```python
from build123d import *

# Parameters (mm, degrees)
CYLINDER1054_R           = 1
CYLINDER1054_DEPTH       = 5
CYLINDER1055_R           = 1
CYLINDER1055_DEPTH       = 5
BOX258_W                 = 36
BOX258_H                 = 16
BOX258_DEPTH             = 1.5
PAD042_DEPTH             = 3
CLONE020_PLACEMENT_ANGLE = -90


with BuildPart() as cylinder1062:
    # Cylinder1054 → Cylinder1054 (new body)
    with BuildSketch(Plane(origin=(33, 3, 0), x_dir=(1, 0, 0), z_dir=(0, 0, 1))):
        Circle(CYLINDER1054_R)
    extrude(amount=CYLINDER1054_DEPTH)


with BuildPart() as fusion151:
    # Cylinder1055 → Cylinder1055 (new body)
    with BuildSketch(Plane(origin=(33, 13, 0), x_dir=(1, 0, 0), z_dir=(0, 0, 1))):
        Circle(CYLINDER1055_R)
    extrude(amount=CYLINDER1055_DEPTH)

    # Fusion151: union Cylinder1062
    add(cylinder1062.part)


with BuildPart() as cut:
    # Box258 → Box258 (new body)
    with BuildSketch(Plane.XY):
        with Locations((18, 8)):
            Rectangle(BOX258_W, BOX258_H)
    extrude(amount=BOX258_DEPTH)

    # Cut: cut Fusion151
    add(fusion151.part, mode=Mode.SUBTRACT)


with BuildPart() as obj1:
    # Sketch067 → Pad042 (new body, symmetric)
    with BuildSketch(Plane(origin=(13, 8, 1.5), x_dir=(0, 0, 1), z_dir=(0, -1, 0))):
        Polygon((0, 0), (10, 0), (10, 3.8), (1.85, 3.8), (1.85, 8.8), (10, 8.8), (10, 12.6), (0, 12.6), align=None)
    extrude(amount=PAD042_DEPTH, both=True)

    # Fusion152: union Cut
    add(cut.part)


with BuildPart() as obj1_1:
    # Clone020 placement: moved
    add(obj1.part.moved(Location((-8, 61.0689, 26.1))).rotate(Axis((-8, 61.0689, 26.1), (0, 0, 1)), CLONE020_PLACEMENT_ANGLE))


solid = obj1_1.part
```
Work out the finished part from the listing and answer in its coordinate system (mm). A direction names the side the tool comes from. Coordinates: 2 decimals unless noted, no trailing zeros. Loops run counter-clockwise (first coordinate to the right, second up) from the corner with the lowest first, then second, coordinate; pieces in that order, holes last. Notation, with made-up numbers: (39.5, -5) - (70.5, -5) arc R23 ccw to (70.5, 24) - close; hole circle Ø3 at (2.25, -37). An arc over 180 degrees is marked (long way). Use a Markdown table: item, result.
Item 1: Find section D-D, the plane y = 57.5. Determine the outline of the cut face in (x, z), and give its area (3 significant figures).
Evaluation:
| item | result |
|---|---|
| outline | (-8, 26.1) - (8, 26.1) - (8, 27.6) - (3, 27.6) - (3, 37.6) - (-3, 37.6) - (-3, 27.6) - (-8, 27.6) - close |
| area | 84.0 mm2 |
Item 2: Find section A-A, the plane z = 31.25. Determine the outline of the cut face in (x, y).
Evaluation:
| item | result |
|---|---|
| outline | (-3, 48.07) - (3, 48.07) - (3, 51.87) - (-3, 51.87) - close; (-3, 56.87) - (3, 56.87) - (3, 60.67) - (-3, 60.67) - close |
Item 3: Given pin 1 Ø3 at (x, z) = (1.5, 31.5) entering from -Y; pin 2 Ø2.5 at (x, y) = (-5, 28.07) entering from +Z; pin 3 Ø3 at (x, z) = (-0.5, 34) entering from +Y; pin 4 Ø4 at (x, y) = (-0.5, 55.5) entering from +Z, each flat-ended and moving along its own axis, determine where each tip first touches the part or whether it passes through.
Evaluation:
| item | result |
|---|---|
| pin 1 | stops at y = 48.07 |
| pin 2 | stops at z = 27.6 |
| pin 3 | stops at y = 60.67 |
| pin 4 | stops at z = 37.6 |
Item 4: The mould has two halves that part along Y. Classify faces 5 (the flat face through (0, 54, 29.45)), 6 (the flat face through (8, 43, 27)), 7 (the flat face through (0, 60.669, 33)), 8 (the cylindrical face through (5.04, 29.07, 26.84)): +Y half, -Y half, draft (parallel to the pull), parting line (faces both ways), or undercut.
Evaluation:
| item | result |
|---|---|
| face 5 | undercut |
| face 6 | draft |
| face 7 | +Y half |
| face 8 | undercut |
Item 5: Find section B-B, the plane x = -5. Determine the outline of the cut face in (y, z), and give its area (3 significant figures).
Evaluation:
| item | result |
|---|---|
| outline | (25.07, 26.1) - (27.07, 26.1) - (27.07, 27.6) - (25.07, 27.6) - close; (29.07, 26.1) - (61.07, 26.1) - (61.07, 27.6) - (29.07, 27.6) - close |
| area | 51.0 mm2 |
Item 6: Find section C-C, the plane y = 28. Determine the outline of the cut face in (x, z).
Evaluation:
| item | result |
|---|---|
| outline | (-8, 26.1) - (-6, 26.1) - (-6, 27.6) - (-8, 27.6) - close; (-4, 26.1) - (4, 26.1) - (4, 27.6) - (-4, 27.6) - close; (6, 26.1) - (8, 26.1) - (8, 27.6) - (6, 27.6) - close |
Item 7: For faces 1 (the flat face through (3, 51.7, 32.5)), 2 (the flat face through (0, 48.069, 33)), 3 (the flat face through (-3, 51.7, 32.5)), 4 (the flat face through (0, 56.869, 33)), determine the directions among +Z, -Z, +X, -X, +Y, -Y from which every point of the face is accessible in a straight line to the end or side of a thin tool.
Evaluation:
| item | result |
|---|---|
| face 1 | +Z, +X, +Y, -Y |
| face 2 | +Z, +X, -X, -Y |
| face 3 | +Z, -X, +Y, -Y |
| face 4 | +Z, +X, -X |
Item 8: Consider probe 1 along Y at (x, z) = (-2.5, 33); probe 2 along Z at (x, y) = (-4, 50); probe 3 along Z at (x, y) = (1, 56.5). Determine where each line is inside the solid, lowest interval first. Write a range as from..to.
Evaluation:
| item | result |
|---|---|
| probe 1 | y = 48.07..51.87, 56.87..60.67 |
| probe 2 | z = 26.1..27.6 |
| probe 3 | z = 26.1..29.45 |
